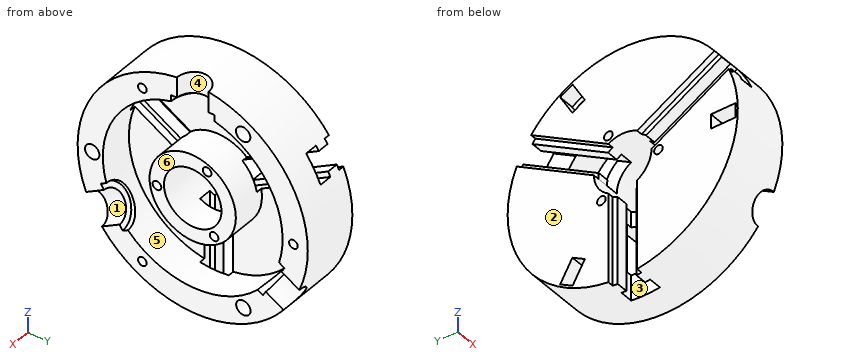
```python
from build123d import *

# Parameters (mm, degrees)
CUT_EXTRUDE1_DEPTH = 81
CIRPATTERN1_COUNT  = 3
CUT_EXTRUDE2_START = -11
SKETCH5_R          = 5
CUT_EXTRUDE2_DEPTH = 30
SKETCH9_R          = 2.999999999
CUT_EXTRUDE3_DEPTH = 41
CIRPATTERN3_COUNT  = 3
SKETCH11_R         = 11
CUT_EXTRUDE4_DEPTH = 15
CUT_EXTRUDE5_START = -4.326695
SKETCH12_R         = 15
CUT_EXTRUDE5_DEPTH = 4.326695
SKETCH15_W         = 10
SKETCH15_H         = 17
CUT_EXTRUDE9_DEPTH = 15
CIRPATTERN5_COUNT  = 3
CIRPATTERN7_COUNT  = 3
CIRPATTERN8_COUNT  = 3


with BuildPart() as part:
    # Sketch1 → Revolve1 (revolve)
    with BuildSketch(Plane.XY):
        Polygon((0, 20), (0, 80), (41, 80), (41, 62.5), (17, 62.5), (17, 30), (41, 30), (41, 20), align=None)
    revolve(axis=Axis((-1000, 0, 0), (1, 0, 0)))

    # Sketch3 → Cut-Extrude1 (cut, through all)
    with BuildSketch(Plane.XY):
        Polygon((0, -10), (0, 10), (4, 10), (4, 6.5), (12, 6.5), (12, 10), (21, 10), (21, -10), (12, -10), (12, -6.5), (4, -6.5), (4, -10), align=None)
    cut_extrude1 = extrude(amount=-CUT_EXTRUDE1_DEPTH, mode=Mode.SUBTRACT)

    # CirPattern1: Cut-Extrude1 ×3 about axis
    cirpattern1_axis = Axis((0, 0, 0), (1, 0, 0))
    for i in range(1, CIRPATTERN1_COUNT):
        add(cut_extrude1.rotate(cirpattern1_axis, i * 360 / CIRPATTERN1_COUNT), mode=Mode.SUBTRACT)

    # Sketch5 → Cut-Extrude2 (cut)
    with BuildSketch(Plane.ZY.offset(CUT_EXTRUDE2_START)):
        with Locations((0, -69.861084208)):
            Circle(SKETCH5_R)
        with Locations((-60.501612866, 35.208201697)):
            Circle(SKETCH5_R)
        with Locations((60.741864319, 35.069492456)):
            Circle(SKETCH5_R)
    extrude(amount=-CUT_EXTRUDE2_DEPTH, mode=Mode.SUBTRACT)

    # Sketch9 → Cut-Extrude3 (cut)
    with BuildSketch(Plane.ZY):
        with Locations((-20.116693275, 14.843134833)):
            Circle(SKETCH9_R)
    cut_extrude3 = extrude(amount=-CUT_EXTRUDE3_DEPTH, mode=Mode.SUBTRACT)

    # CirPattern3: Cut-Extrude3 ×3 about axis
    cirpattern3_axis = Axis((0, 0, 0), (1, 0, 0))
    for i in range(1, CIRPATTERN3_COUNT):
        add(cut_extrude3.rotate(cirpattern3_axis, i * 360 / CIRPATTERN3_COUNT), mode=Mode.SUBTRACT)

    # Sketch11 → Cut-Extrude4 (cut)
    with BuildSketch(Plane.XY.offset(80)):
        with Locations((41, 0)):
            Circle(SKETCH11_R)
    cut_extrude4 = extrude(amount=-CUT_EXTRUDE4_DEPTH, mode=Mode.SUBTRACT)

    # Sketch12 → Cut-Extrude5 (cut)
    with BuildSketch(Plane.XY.offset(65).offset(CUT_EXTRUDE5_START)):
        with Locations((41, 0)):
            Circle(SKETCH12_R)
    cut_extrude5 = extrude(amount=CUT_EXTRUDE5_DEPTH, mode=Mode.SUBTRACT)

    # Sketch15 → Cut-Extrude9 (cut)
    with BuildSketch(Plane(origin=(11, 0, 0), x_dir=(0, 0, -1), z_dir=(1, 0, 0))):
        with Locations((0, -69.861084208)):
            Rectangle(SKETCH15_W, SKETCH15_H)
    cut_extrude9 = extrude(amount=-CUT_EXTRUDE9_DEPTH, mode=Mode.SUBTRACT)

    # CirPattern5: Cut-Extrude9 ×3 about axis
    cirpattern5_axis = Axis((0, 0, 0), (1, 0, 0))
    for i in range(1, CIRPATTERN5_COUNT):
        add(cut_extrude9.rotate(cirpattern5_axis, i * 360 / CIRPATTERN5_COUNT), mode=Mode.SUBTRACT)

    # Sketch19 → Ø6.0mm Dowel Hole3 (revolve, cut)
    with BuildSketch(Plane(origin=(41, 70, 0), x_dir=(0, 0, -1), z_dir=(0, 1, 0))):
        Polygon((0, 0), (0, 31.802581857), (3, 30), (3, 0), align=None)
    f_6_0mm_dowel_hole3 = revolve(axis=Axis((47.35, 70, 0), (-1, 0, 0)), mode=Mode.SUBTRACT)

    # CirPattern7: Ø6.0mm Dowel Hole3 ×3 about axis
    cirpattern7_axis = Axis((0, 0, 0), (1, 0, 0))
    for i in range(1, CIRPATTERN7_COUNT):
        add(f_6_0mm_dowel_hole3.rotate(cirpattern7_axis, i * 360 / CIRPATTERN7_COUNT), mode=Mode.SUBTRACT)

    # CirPattern8: Cut-Extrude4, Cut-Extrude5 ×3 about axis
    cirpattern8_axis = Axis((0, 0, 0), (1, 0, 0))
    for i in range(1, CIRPATTERN8_COUNT):
        add(cut_extrude4.rotate(cirpattern8_axis, i * 360 / CIRPATTERN8_COUNT), mode=Mode.SUBTRACT)
        add(cut_extrude5.rotate(cirpattern8_axis, i * 360 / CIRPATTERN8_COUNT), mode=Mode.SUBTRACT)


solid = part.part
```
Could you check a few things on this model? Use its own coordinates, in mm. Face numbers are marked on the shaded views. A direction names the side the tool comes from. Coordinates: 2 decimals unless noted, no trailing zeros. Write each loop counter-clockwise with the first axis right and the second up, starting at its lowest first coordinate (ties: lowest second). Pieces come first, ordered by that corner, then holes. Notation, with made-up numbers: (77, 61) -> (111, 61) arc R13 cw to (111, 66) -> close; hole circle Ø9 at (59, 37.25). An arc over 180 degrees is marked (long way). Write item = value, one per line. Start each with the question number.
(1) I want a section at A-A (y = 0). Please give me the cut outline in (x, z).
(2) I want a section at C-C (x = 35.5). Give the number of separate pieces and of enclosed holes in the cut face, plus the area to 3 significant figures.
(3) We'd pull the mould along X, two halves only. Please class the marked faces 1, 2 and 3: released by +X, released by -X, zero draft, split by the parting line, or undercut.
(4) I want a section at B-B (z = 11). Please give me the cut outline in (x, y), plus the area to 3 significant figures.
(5) Which directions (+Z, -Z, +X, -X, +Y, -Y) give clear straight access to the entire face, cutting with the end or side of a thin tool? Please do the marked faces 4, 5 and 6.
(6) I need wall thicknesses on line 1 (Y direction, x = 36, z = 24.5); line 2 (Y direction, x = 36, z = 12.5); line 3 (Z direction, x = 10.5, y = 15.5). Which ranges of each line are inside material? Lowest first, please. Write a range as [from, to].
(7) Will these pins go through, and if not, where does the flat tip stop? pin 1 (1.8 mm diameter, centred on y = -9, z = -34.5, fed in from -X); pin 2 (3.5 mm diameter, centred on y = 10, z = 22.91, fed in from +X); pin 3 (3 mm diameter, centred on x = 32, y = -62, fed in from +Z); pin 4 (11 mm diameter, centred on x = 4.5, z = 0, fed in from -Y).
Result set:
q1.outline = (0, 20) -> (41, 20) -> (41, 30) -> (17, 30) -> (17, 62.5) -> (26, 62.5) -> (26, 65) -> (30, 65) -> (30, 80) -> (0, 80) -> close; (21, -80) -> (41, -80) -> (41, -62.5) -> (21, -62.5) -> close; (21, -30) -> (41, -30) -> (41, -20) -> (21, -20) -> close
q2.separate_pieces = 4
q2.enclosed_holes = 10
q2.area = 7,900 mm2
q3.face_1 = released by +X
q3.face_2 = released by -X
q3.face_3 = undercut
q4.outline = (0, -79.24) -> (41, -79.24) -> (41, -61.52) -> (17, -61.52) -> (17, -39.05) -> (12, -39.05) -> (12, -32.05) -> (4, -32.05) -> (4, -39.05) -> (0, -39.05) -> close; (0, 39.05) -> (4, 39.05) -> (4, 32.05) -> (12, 32.05) -> (12, 39.05) -> (17, 39.05) -> (17, 61.52) -> (41, 61.52) -> (41, 79.24) -> (0, 79.24) -> close; (21, -27.91) -> (41, -27.91) -> (41, -16.7) -> (21, -16.7) -> close; (21, 16.7) -> (41, 16.7) -> (41, 27.91) -> (21, 27.91) -> close
q4.area = 2,780 mm2
q5.face_4 = +Z, +X
q5.face_5 = +X
q5.face_6 = +Z, -Z, +X, +Y, -Y
q6.line_1 = [-76.16, -57.5], [-17.31, 7.45], [12.55, 17.31], [57.5, 76.16]
q6.line_2 = [-79.02, -61.24], [-27.27, -15.61], [15.61, 27.27], [61.24, 79.02]
q6.line_3 = [-78.48, -23.04], [-17.19, -12.64], [16.45, 78.48]
q7.pin_1 = 4
q7.pin_2 = through
q7.pin_3 = 52.34
q7.pin_4 = -80
